Here's how the part is built. I have some questions about the finished solid (model axes, mm). A direction names the side the tool comes from. Coordinates: 2 decimals unless noted, no trailing zeros. Write each loop counter-clockwise with the first axis right and the second up, starting at its lowest first coordinate (ties: lowest second). Pieces come first, ordered by that corner, then holes. Notation, with made-up numbers: M -9.5,-13 L 2.5,-13 A16 ccw 2.5,7 Z; hole C 85.5,26 d8. An arc over 180 degrees is marked long. Use one line per item in the form item = value. Start each with the question number.
1. Please list where these lines run through material, in increasing order: line 1 along Y through (x, z) = (-36, -5.75); line 2 along Z through (x, y) = (101.5, -234); line 3 along Y through (x, z) = (-69.5, -0.75). Write a range as [from, to].
2. I want a section at A-A, the plane x = 84. List the corners of the cut face in (y, z) for me.
3. I'm going to push flat-ended pins straight in: pin 1 Ø0.6 at (x, z) = (-39.5, -0.5) entering from -Y; pin 2 Ø0.6 at (x, z) = (54.5, -1) entering from +Y. Where does each tip first touch, or does it pass through?
4. I want a section at B-B, the plane y = -159. List the corners of the cut face in (x, z) for me, plus the area to 3 significant figures.
5. I want a section at C-C, the plane z = 2.75. List the corners of the cut face in (x, y) for me.
6. On a 3-axis mill with a long thin cutter (end or side, diameter ignored), from which of +Z, -Z, +X, -X, +Y, -Y can I reach the whole of each face in a straight line? I mean faces 1 (the face through (-2, -160, 0)), 2 (the face through (-2, -220, -2)), 3 (the face through (1, -230.386, -7)). Say none if no direction works.
7. Thinking about a two-plate mould opening in X: for faces 4 (the face through (-141, -189, -1)), 5 (the face through (1, -220.386, -7)), 6 (the face through (105, -225, 5)), 7 (the face through (-2, -220, 0)), which applies, released by +X, released by -X, zero draft, split by the parting line, or undercut?
from build123d import *

# Parameters (mm, degrees)
BOSS_EXTRUDE1_DEPTH            = 141
BOSS_EXTRUDE1_DEPTH_BACK       = 141
SKETCH1_W                      = 22
SKETCH1_H                      = 100
CAVITY1_START                  = -2
CAVITY1_OUTLINE_W              = 282
CAVITY1_OUTLINE_H              = 40
CAVITY1_DEPTH                  = 2
CUT_EXTRUDE1_REACH             = 280.613
SKETCH2_W                      = 210
SKETCH2_H                      = 10
CUT_EXTRUDE1_DIRECTION_2_REACH = 280.613


# Read off the part's stored shape, not the designer's step: Cavity1
with BuildPart() as part:
    # Sketch1 → Boss-Extrude1 (new, two sides: drawn at the far end of the back side and taken through both)
    with BuildSketch(Plane(origin=(0, 0, 0), x_dir=(0, 0, -1), z_dir=(1, 0, 0)).offset(-BOSS_EXTRUDE1_DEPTH_BACK)):
        with Locations((1, -190)):
            Rectangle(SKETCH1_W, SKETCH1_H)
    extrude(amount=BOSS_EXTRUDE1_DEPTH + BOSS_EXTRUDE1_DEPTH_BACK)

    # Cavity1 outline → Cavity1 (cut)
    with BuildSketch(Plane.XY.offset(CAVITY1_START)):
        with Locations((0, -160)):
            Rectangle(CAVITY1_OUTLINE_W, CAVITY1_OUTLINE_H)
    cavity1 = extrude(amount=CAVITY1_DEPTH, mode=Mode.SUBTRACT)

    # Mirror1: Cavity1 across plane
    add(cavity1.mirror(Plane.ZX.offset(-190)), mode=Mode.SUBTRACT)

    # Cut-Extrude1: up to this face of the body (flat: up to its plane)
    cut_extrude1_end = Plane(part.part.faces().sort_by_distance((0, -190, 10))[0])
    # Sketch2 → Cut-Extrude1 (cut, up to the picked face)
    with BuildSketch(Plane(origin=(0, 0, 0), x_dir=(-1, 0, 0), z_dir=(0, 0, -1)), mode=Mode.PRIVATE) as cut_extrude1_sk1:
        with Locations((0, -225.386342941)):
            Rectangle(SKETCH2_W, SKETCH2_H)
    cut_extrude1_tool1 = split(extrude(cut_extrude1_sk1.sketch, amount=-CUT_EXTRUDE1_REACH, mode=Mode.PRIVATE), bisect_by=cut_extrude1_end, keep=Keep.BOTH, mode=Mode.PRIVATE)
    add(cut_extrude1_tool1.solids().sort_by(Axis((0, -225.386343, 0), (0, 0, 1)))[0], mode=Mode.SUBTRACT)

    # Cut-Extrude1 direction 2: up to this face of the body (flat: up to its plane)
    cut_extrude1_direction_2_end = Plane(part.part.faces().sort_by_distance((0, -190, -12))[0])
    # Sketch2 → Cut-Extrude1 direction 2 (cut, up to the picked face)
    with BuildSketch(Plane(origin=(0, 0, 0), x_dir=(-1, 0, 0), z_dir=(0, 0, -1)), mode=Mode.PRIVATE) as cut_extrude1_direction_2_sk1:
        with Locations((0, -225.386342941)):
            Rectangle(SKETCH2_W, SKETCH2_H)
    cut_extrude1_direction_2_tool1 = split(extrude(cut_extrude1_direction_2_sk1.sketch, amount=CUT_EXTRUDE1_DIRECTION_2_REACH, mode=Mode.PRIVATE), bisect_by=cut_extrude1_direction_2_end, keep=Keep.BOTH, mode=Mode.PRIVATE)
    add(cut_extrude1_direction_2_tool1.solids().sort_by(Axis((0, -225.386343, 0), (0, 0, -1)))[0], mode=Mode.SUBTRACT)


solid = part.part
Answer list:
q1.line_1 = [-240, -230.39], [-220.39, -140]
q1.line_2 = [-12, -2], [0, 10]
q1.line_3 = [-200, -180]
q2.outline = M -240,-12 L -230.39,-12 L -230.39,-2 L -240,-2 Z; M -240,0 L -230.39,0 L -230.39,10 L -240,10 Z; M -220.39,-12 L -140,-12 L -140,-2 L -180,-2 L -180,0 L -140,0 L -140,10 L -220.39,10 L -220.39,0 L -200,0 L -200,-2 L -220.39,-2 Z
q3.pin_1 = -200
q3.pin_2 = -180
q4.outline = M -141,-12 L 141,-12 L 141,-2 L -141,-2 Z; M -141,0 L 141,0 L 141,10 L -141,10 Z
q4.area = 5,640 mm²
q5.outline = M -141,-240 L 141,-240 L 141,-140 L -141,-140 Z; hole M -105,-230.39 L 105,-230.39 L 105,-220.39 L -105,-220.39 Z
q6.face_1 = +X, -X, +Y
q6.face_2 = +X, -X, -Y
q6.face_3 = +Z, -Z
q7.face_4 = released by -X
q7.face_5 = undercut
q7.face_6 = undercut
q7.face_7 = zero draft
